Verification items for the finished model (mm, model axes). Coordinates: 2 decimals unless noted, no trailing zeros. Write each loop counter-clockwise with the first axis right and the second up, starting at its lowest first coordinate (ties: lowest second). Pieces come first, ordered by that corner, then holes. Notation, with made-up numbers: M -36.5,28 L -13.5,28 A10 ccw -13.5,46 Z; hole C 59.5,25 d6. An arc over 180 degrees is marked long. Answer in a Markdown table with one row per item.
from build123d import *

# Parameters (mm, degrees)
F1_DEPTH = 5
F2_SIZE  = 4.99999


# Not quite as in the source:
# - a fillet or chamfer is up to 0.001 mm smaller than in the source, because OpenCascade refuses the exact size


with BuildPart() as f1:
    # F0 (on Top) → F1 (new body)
    with BuildSketch(Plane.XY):
        Polygon((-27.5, -52.5), (27.5, -52.5), (27.5, -14.74), (-27.5, -11.5), align=None)
        Polygon((-27.5, -11.5), (27.5, -14.74), (27.5, -11.5), align=None)
    extrude(amount=F1_DEPTH)

    # F2 (size 5 in the source; OpenCascade refuses exactly that, so slightly less here)
    f2_edges = [f1.edges().sort_by_distance(p)[0] for p in [
        (-27.5, -32, 0),
        (0, -52.5, 0),
        (27.5, -32, 0),
    ]]
    chamfer(f2_edges, length=F2_SIZE)


solid = f1.part
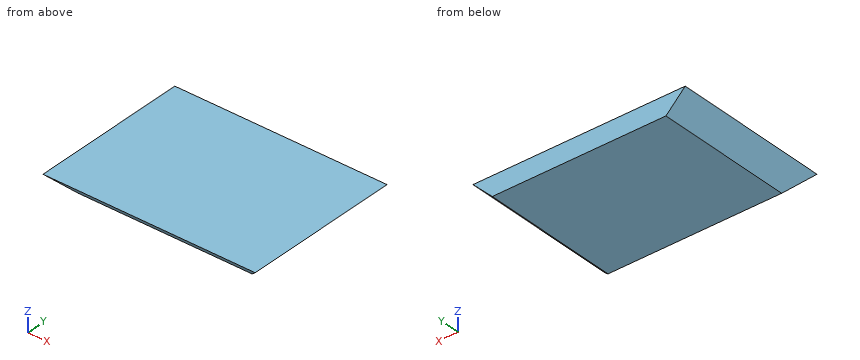
1) Depth check by flat-ended pin: pin 1 (1 mm diameter, centred on y = -18, z = 1, fed in from -X). Enter the tip coordinate at first touch or a pass-through.
Response values:
| item | result |
|---|---|
| pin 1 | stops at x = -24 |
2) Sectioned sample at C-C (z = 2). Record the cut outline in (x, y), then the cut area to 3 significant figures.
Response values:
| item | result |
|---|---|
| outline | M -24.5,-49.5 L 24.5,-49.5 L 24.5,-11.5 L -24.5,-11.5 Z |
| area | 1,860 mm² |
3) Thickness scan on L1, parallel to X at y = -44, z = 2.05; L2, parallel to Y at x = -3.5, z = 3.15; L3, parallel to Y at x = 18.5, z = 1.25. Record the ranges inside material, lowest first. Write a range as [from, to].
Response values:
| item | result |
|---|---|
| L1 | x = [-24.55, 24.55] |
| L2 | y = [-50.65, -11.5] |
| L3 | y = [-48.75, -11.5] |
